Source: CAD feature listing. Evaluate the final solid. Frame: model axes, mm. Coordinates: 2 decimals unless noted, no trailing zeros. Order: outer loops, then holes, each group sorted by start corner. A loop starts at its lowest first (then second) coordinate and runs counter-clockwise, first axis right, second up.
Autodesk Inventor part; units mm, degrees
ref_plane "YZ Plane" through (0, 0, 0) normal (1, 0, 0) x (0, 1, 0)
ref_plane "XZ Plane" through (0, 0, 0) normal (0, 1, 0) x (-1, 0, 0)
ref_plane "XY Plane" through (0, 0, 0) normal (0, 0, 1) x (1, 0, 0)
sketch "Sketch1" plane through (0, 0, 0) normal (0, 1, 0) x (-1, 0, 0)
  line L0 (-7.25, 7.25) -> (7.25, 7.25)
  line L1 (7.25, 7.25) -> (7.25, -7.25)
  line L2 (7.25, -7.25) -> (-7.25, -7.25)
  line L3 (-7.25, -7.25) -> (-7.25, 7.25)
  line L4 (-7.25, 7.25) -> (7.25, -7.25) construction
  line L5 (7.25, 7.25) -> (-7.25, -7.25) construction
  point P0 (0, 0)
  dimension "d0" = 14.5
  dimension "d1" = 14.5
extrude "Extrusion1" add sketch "Sketch1" along normal blind 76.2
sketch "Sketch2" plane through (0, 76.2, 0) normal (0, 1, 0) x (1, 0, 0)
  line L0 (10, -10) -> (-10, -10)
  line L1 (-10, -10) -> (-10, 10)
  line L2 (-10, 10) -> (10, 10)
  line L3 (10, 10) -> (10, -10)
  line L4 (10, -10) -> (-10, 10) construction
  line L5 (-10, -10) -> (10, 10) construction
  point P0 (0, 0)
  dimension "d4" = 20
  dimension "d5" = 20
extrude "Extrusion2" add sketch "Sketch2" along normal blind 5
sketch "Sketch3" plane through (0, 81.2, 0) normal (0, 1, 0) x (1, 0, 0)
  line L0 (7.5, -7.5) -> (-7.5, -7.5)
  line L1 (-7.5, -7.5) -> (-7.5, 7.5)
  line L2 (-7.5, 7.5) -> (7.5, 7.5)
  line L3 (7.5, 7.5) -> (7.5, -7.5)
  line L4 (7.5, -7.5) -> (-7.5, 7.5) construction
  line L5 (-7.5, -7.5) -> (7.5, 7.5) construction
  line L6 (10, -10) -> (-10, -10)
  line L7 (-10, -10) -> (-10, 10)
  line L8 (-10, 10) -> (10, 10)
  line L9 (10, 10) -> (10, -10)
  line L10 (10, -10) -> (-10, 10) construction
  line L11 (-10, -10) -> (10, 10) construction
  point P0 (0, 0)
  dimension "d8" = 15
  dimension "d9" = 15
extrude "Extrusion3" add sketch "Sketch3" along normal blind 76.2
sketch "Sketch4" plane through (10, 76.2, 10) normal (1, 0, 0) x (0, 0, -1)
  line L0 (20, 0) -> (20, 81.2)
  line L1 (15, 81.2) -> (15, 0)
  line L2 (0, 0) -> (20, 0)
  line L3 (15, 81.2) -> (13, 81.2)
  line L4 (17.5, 81.2) -> (2.5, 81.2)
  line L5 (13, 81.2) -> (13, 0)
  line L6 (13, 0) -> (15, 0)
  line L7 (20, 81.2) -> (0, 81.2)
  point P0 (10, -76.2)
  dimension "d12" = 2
extrude "Extrusion4" add sketch "Sketch4" along normal blind 10 contours L2 L5 L3 L1
sketch "Sketch5" plane through (10, 76.2, -3) normal (0, 0, 1) x (1, 0, 0)
  line L0 (0, 81.2) -> (10, 81.2)
  line L1 (10, 81.2) -> (8, 81.2)
  line L2 (8, 81.2) -> (8, 0)
  line L3 (8, 0) -> (10, 0)
  line L4 (10, 0) -> (10, 81.2)
  point P0 (-10, -76.2)
  dimension "d15" = 2
extrude "Extrusion5" add sketch "Sketch5" along normal blind 8
sketch "Sketch6" plane through (20, 76.2, 10) normal (1, 0, 0) x (0, 0, -1)
  line L0 (5, 81.2) -> (3, 81.2)
  line L1 (3, 81.2) -> (3, 0)
  line L2 (3, 0) -> (5, 0)
  line L3 (5, 0) -> (5, 81.2)
  point P0 (10, -76.2)
  dimension "d18" = 2
extrude "Extrusion6" add sketch "Sketch6" against normal blind 4
sketch "Sketch7" plane through (0, 76.2, 0) normal (0, -1, 0) x (1, 0, 0)
  line L0 (10, -5) -> (20, -5)
  line L1 (20, -5) -> (20, 7)
  line L2 (20, 7) -> (10, 7)
  line L3 (10, 7) -> (10, -5)
  point P0 (0, 0)
extrude "Extrusion7" cut sketch "Sketch7" against normal through all
sketch "Sketch8" plane through (7.25, 0, -7.25) normal (0, 0, -1) x (-1, 0, 0)
  line L0 (0, 0) -> (0, 76.2)
  line L1 (0, 0) -> (0, 76.2)
  line L2 (0, 38.1) -> (14.5, 38.1)
  line L3 (14.5, 38.1) -> (14.5, 0)
  line L4 (14.5, 0) -> (0, 0)
  line L5 (0, 0) -> (0, 38.1)
  point P0 (7.25, 0)
extrude "Extrusion8" cut sketch "Sketch8" against normal through all
sketch "Sketch9" plane through (10, 76.2, -10) normal (0, 0, -1) x (-1, 0, 0)
  line L0 (0, 0) -> (0, 20)
  line L1 (0, 0) -> (0, 81.2)
  line L2 (0, 20) -> (20, 20)
  line L3 (20, 20) -> (20, 81.2)
  line L4 (20, 81.2) -> (0, 81.2)
  line L5 (0, 81.2) -> (0, 20)
  point P0 (10, -76.2)
  dimension "d25" = 20
extrude "Extrusion9" cut sketch "Sketch9" against normal through all
sketch "Sketch10" plane through (-10, 96.2, -10) normal (0, 1, 0) x (1, 0, 0)
  line L0 (17.5, -2.5) -> (2.5, -2.5)
  line L1 (2.5, -2.5) -> (2.5, -17.5)
  line L2 (2.5, -17.5) -> (17.5, -17.5)
  line L3 (17.5, -17.5) -> (17.5, -2.5)
  point P0 (10, -10)
extrude "Extrusion10" add sketch "Sketch10" against normal blind 15
sketch "Sketch12" plane through (10, 76.2, 10) normal (1, 0, 0) x (0, 0, -1)
  line L0 (20, 20) -> (9, 20)
  line L1 (20, 20) -> (0, 20)
  line L2 (2.75, 0) -> (17.25, 0)
  line L3 (20, 20) -> (13, 20)
  line L4 (13, 20) -> (13, 0)
  line L5 (13, 0) -> (20, 0)
  line L6 (20, 0) -> (20, 20)
  point P0 (10, -76.2)
  dimension "d30" = 11
  dimension "d31" = 7
extrude "Extrusion11" add sketch "Sketch12" along normal blind 10
sketch "Sketch13" plane through (-10, 76.2, -10) normal (0, 0, -1) x (-1, 0, 0)
  line L0 (-17.25, 0) -> (-17.25, 20)
  line L1 (0, 20) -> (-30, 20)
  line L2 (-17.25, -38.1) -> (-17.25, 0)
  line L3 (-20, 0) -> (-20, 20)
  line L4 (-20, 0) -> (-20, 20)
  line L5 (-20, 10) -> (-24, 10)
  circle A0 centre (-24, 10) radius 1.4
  point P0 (-10, -76.2)
  dimension "d34" = 4
  dimension "d35" = 2.8
extrude "Extrusion12" cut sketch "Sketch13" against normal through all
sketch "Sketch14" plane through (-10, 76.2, 10) normal (0, 0, 1) x (1, 0, 0)
  line L0 (20, 20) -> (-2.0792, 20)
  line L1 (-2.0792, 20) -> (-2.0792, -41.5278)
  line L2 (-2.0792, -41.5278) -> (20, -41.5278)
  line L3 (20, -41.5278) -> (20, 20)
  point P0 (10, -76.2)
extrude "Extrusion13" cut sketch "Sketch14" against normal through all
properties part number "NailBitHold"
Q1. Section query B-B on x = 14. Output: boundary loops of the cut face in (y, z).
Solutions:
outline: (76.2, -10) - (84.8, -10) - (84.8, -3) - (76.2, -3) - close; (87.6, -10) - (96.2, -10) - (96.2, -3) - (87.6, -3) - close
Q2. Material intervals for line 1 along X through (y, z) = (86.2, -4.75); line 2 along Y through (x, z) = (14, -8); line 3 along Y through (x, z) = (13, -7.25), sorted ascending.
Solutions:
line 1: x = 10 to 12.6, 15.4 to 20
line 2: y = 76.2 to 84.8, 87.6 to 96.2
line 3: y = 76.2 to 85.22, 87.18 to 96.2
Q3. Pin query (flat end, axial travel): P1, Ø3.5, axis at x = 14, y = 86.2, coming from the +Z side. Return the tip coordinate at first contact, or that it passes through.
Solutions:
P1: stops at z = -3
Q4. Section query A-A on y = 86.2. Output: boundary loops of the cut face in (x, z).
Solutions:
outline: (10, -10) - (12.6, -10) - (12.6, -3) - (10, -3) - close; (15.4, -10) - (20, -10) - (20, -3) - (15.4, -3) - close
Q5. Section query C-C on z = -6.5. Output: boundary loops of the cut face in (x, y), plus the area to 3 significant figures.
Solutions:
outline: (10, 76.2) - (20, 76.2) - (20, 96.2) - (10, 96.2) - close; hole circle Ø2.8 at (14, 86.2)
area: 194 mm2
Q6. Pull-direction query (Y, two-part tool) for faces 1 (the cylindrical face through (14.18, 87.59, -6.55)), 2 (the flat face through (15, 96.2, -7)), 3 (the flat face through (16, 86, -10)); classes: pulls with the +Y half, pulls with the -Y half, needs draft (parallel to the pull), parting line crosses it, or undercut.
Solutions:
face 1: undercut
face 2: pulls with the +Y half
face 3: needs draft
